```python
from build123d import *

# Parameters (mm, degrees)
SKETCH1_R               = 14.7
SKETCH1_R_2             = 13.4
BOSS_EXTRUDE1_DEPTH     = 7
SKETCH2_W               = 1.6
SKETCH2_H               = 2
BOSS_EXTRUDE2_DEPTH     = 7
CUT_EXTRUDE1_DEPTH      = 22.935815462
CUT_EXTRUDE1_DEPTH_BACK = 22.935815462
SKETCH3_R               = 1.1
SKETCH4_R               = 17.05
SKETCH4_R_2             = 11.5
BOSS_EXTRUDE3_DEPTH     = 2
BOSS_EXTRUDE4_DEPTH     = 2
CUT_EXTRUDE2_REACH      = 27.108
SKETCH6_R               = 1


with BuildPart() as part:
    # Sketch1 → Boss-Extrude1 (new body)
    with BuildSketch(Plane.XY):
        Circle(SKETCH1_R)
        Circle(SKETCH1_R_2, mode=Mode.SUBTRACT)
    extrude(amount=BOSS_EXTRUDE1_DEPTH)

    # Sketch2 → Boss-Extrude2 (add)
    with BuildSketch(Plane.XY):
        with Locations((0, -12.4)):
            Rectangle(SKETCH2_W, SKETCH2_H)
    extrude(amount=BOSS_EXTRUDE2_DEPTH)

    # Sketch3 → Cut-Extrude1 (cut, two sides: drawn at the far end of the back side and taken through both)
    with BuildSketch(Plane(origin=(0, 0, 0), x_dir=(0, 0, -1), z_dir=(1, 0, 0)).offset(-CUT_EXTRUDE1_DEPTH_BACK)):
        with Locations((-3.67, 0)):
            Circle(SKETCH3_R)
    extrude(amount=CUT_EXTRUDE1_DEPTH + CUT_EXTRUDE1_DEPTH_BACK, mode=Mode.SUBTRACT)

    # Sketch4 → Boss-Extrude3 (add)
    with BuildSketch(Plane.XY):
        Circle(SKETCH4_R)
        Circle(SKETCH4_R_2, mode=Mode.SUBTRACT)
    extrude(amount=-BOSS_EXTRUDE3_DEPTH)

    # Sketch5 → Boss-Extrude4 (add)
    with BuildSketch(Plane.XY):
        with BuildLine():
            Line((-6.5, -3), (-3, -3))
            Line((-3, -3), (-3, -11.5))
            Line((-3, -11.5), (3, -11.5))
            Line((3, -11.5), (3, -3))
            Line((3, -3), (6.5, -3))
            ThreePointArc((6.5, -3), (9.5, 0), (6.5, 3))
            Line((6.5, 3), (3, 3))
            Line((3, 3), (3, 11.5))
            Line((3, 11.5), (0, 11.5))
            Line((0, 11.5), (-3, 11.5))
            Line((-3, 11.5), (-3, 3))
            Line((-3, 3), (-6.5, 3))
            ThreePointArc((-6.5, 3), (-9.5, 0), (-6.5, -3))
        make_face()
    extrude(amount=-BOSS_EXTRUDE4_DEPTH)

    # Sketch6 → Cut-Extrude2 (cut, up to next)
    with BuildSketch(Plane.XY, mode=Mode.PRIVATE) as cut_extrude2_sk1:
        Circle(SKETCH6_R)
    cut_extrude2_tool1 = extrude(cut_extrude2_sk1.sketch, amount=-CUT_EXTRUDE2_REACH, mode=Mode.PRIVATE) & part.part
    # Sketch6 → Cut-Extrude2 (cut, up to next)
    with BuildSketch(Plane.XY, mode=Mode.PRIVATE) as cut_extrude2_sk2:
        with Locations((6.5, 0)):
            Circle(SKETCH6_R)
    cut_extrude2_tool2 = extrude(cut_extrude2_sk2.sketch, amount=-CUT_EXTRUDE2_REACH, mode=Mode.PRIVATE) & part.part
    # Sketch6 → Cut-Extrude2 (cut, up to next)
    with BuildSketch(Plane.XY, mode=Mode.PRIVATE) as cut_extrude2_sk3:
        with Locations((-6.5, 0)):
            Circle(SKETCH6_R)
    cut_extrude2_tool3 = extrude(cut_extrude2_sk3.sketch, amount=-CUT_EXTRUDE2_REACH, mode=Mode.PRIVATE) & part.part
    # Sketch6 → Cut-Extrude2 (cut, up to next)
    with BuildSketch(Plane.XY, mode=Mode.PRIVATE) as cut_extrude2_sk4:
        with Locations((0, 8.5)):
            Circle(SKETCH6_R)
    cut_extrude2_tool4 = extrude(cut_extrude2_sk4.sketch, amount=-CUT_EXTRUDE2_REACH, mode=Mode.PRIVATE) & part.part
    # Sketch6 → Cut-Extrude2 (cut, up to next)
    with BuildSketch(Plane.XY, mode=Mode.PRIVATE) as cut_extrude2_sk5:
        with Locations((0, -8.5)):
            Circle(SKETCH6_R)
    cut_extrude2_tool5 = extrude(cut_extrude2_sk5.sketch, amount=-CUT_EXTRUDE2_REACH, mode=Mode.PRIVATE) & part.part
    add(cut_extrude2_tool1.solids().sort_by_distance((0, 0, 0))[0], mode=Mode.SUBTRACT)
    add(cut_extrude2_tool2.solids().sort_by_distance((6.5, 0, 0))[0], mode=Mode.SUBTRACT)
    add(cut_extrude2_tool3.solids().sort_by_distance((-6.5, 0, 0))[0], mode=Mode.SUBTRACT)
    add(cut_extrude2_tool4.solids().sort_by_distance((0, 8.5, 0))[0], mode=Mode.SUBTRACT)
    add(cut_extrude2_tool5.solids().sort_by_distance((0, -8.5, 0))[0], mode=Mode.SUBTRACT)


solid = part.part
```
Source: CAD feature listing. Evaluate the final solid. Frame: model axes, mm. A direction names the side the tool comes from. Give positions to 0.01 mm unless a question says otherwise; leave off trailing zeros. Loops run counter-clockwise (first coordinate to the right, second up) from the corner with the lowest first, then second, coordinate; pieces in that order, holes last. Notation, with made-up numbers: (51, -33.75) - (64, -33.75) arc R31 ccw to (64, -7.75) - close; hole circle Ø2 at (-14.5, -25). An arc over 180 degrees is marked (long way). Use CSV: the item, a comma, the result in double quotes. Start each with the question number.
1. Section C-C (y = 7). Output: boundary loops of the cut face in (x, z).
2. Section A-A (z = 5.5). Output: boundary loops of the cut face in (x, y), then the cut area to 3 significant figures.
3. Section D-D (z = 3.75). Output: boundary loops of the cut face in (x, y), then the cut area to 3 significant figures.
4. Pin query (flat end, axial travel): pin 1 (8 mm diameter, centred on x = 6, y = 4, fed in from +Z); pin 2 (1.5 mm diameter, centred on y = -7, z = -1, fed in from +X); pin 3 (1.6 mm diameter, centred on y = -12, z = 2.5, fed in from -X). Return the tip coordinate at first contact, or that it passes through.
5. Ray query, L1, parallel to Y at x = 0, z = -0.85; L2, parallel to X at y = 0, z = 2.25; L3, parallel to X at y = -11.5, z = 3.5. Return the intervals inside material, ascending.
6. Section B-B (x = 11). Output: boundary loops of the cut face in (y, z), then the cut area to 3 significant figures.
7. Draft query along Y for faces 1 (the cylindrical face through (5.7, -0.6, -1)), 2 (the cylindrical face through (14.02, 4.42, 3.45)), 3 (the flat face through (0, -13, 7)). Return one class per face: +Y half, -Y half, draft (parallel to the pull), parting line (faces both ways), or undercut.
8. Reachability of faces 4 (the flat face through (3, 7, -1)), 5 (the flat face through (0, -11.4, 3)), 6 (the cylindrical face through (-14.04, 0.33, 2.62)) from +Z, -Z, +X, -X, +Y, -Y: full face, straight path, thin tool, end or side. Return the list, or none.
Response:
1,outline,"(-15.55, -2) - (-9.12, -2) - (-9.12, 0) - (-11.43, 0) - (-11.43, 7) - (-12.93, 7) - (-12.93, 0) - (-15.55, 0) - close; (-3, -2) - (3, -2) - (3, 0) - (-3, 0) - close; (9.12, -2) - (15.55, -2) - (15.55, 0) - (12.93, 0) - (12.93, 7) - (11.43, 7) - (11.43, 0) - (9.12, 0) - close"
2,outline,"circle Ø29.4 at (0, 0); hole (-0.8, -13.38) - (-0.8, -11.4) - (0.8, -11.4) - (0.8, -13.38) arc R13.4 ccw (long way) to start"
2,area,"118 mm²"
3,outline,"(-14.66, -1.1) arc R14.7 ccw to (14.66, -1.1) - (13.36, -1.1) arc R13.4 cw to (0.8, -13.38) - (0.8, -11.4) - (-0.8, -11.4) - (-0.8, -13.38) arc R13.4 cw to (-13.36, -1.1) - close; (-14.66, 1.1) - (-13.36, 1.1) arc R13.4 cw to (13.36, 1.1) - (14.66, 1.1) arc R14.7 ccw to start"
3,area,"112 mm²"
4,pin 1,"z = 0"
4,pin 2,"x = 15.86"
4,pin 3,"x = -9.52"
5,L1,"-17.05 to -9.5, -7.5 to -1, 1 to 7.5, 9.5 to 17.05"
5,L2,"-14.7 to -13.4, 13.4 to 14.7"
5,L3,"-9.16 to -6.88, -0.8 to 0.8, 6.88 to 9.16"
6,outline,"(-13.03, -2) - (-3.35, -2) - (-3.35, 0) - (-7.65, 0) - (-7.65, 7) - (-9.75, 7) - (-9.75, 0) - (-13.03, 0) - close; (3.35, -2) - (13.03, -2) - (13.03, 0) - (9.75, 0) - (9.75, 7) - (7.65, 7) - (7.65, 0) - (3.35, 0) - close"
6,area,"68.1 mm²"
7,face 1,"undercut"
7,face 2,"parting line"
7,face 3,"draft"
8,face 4,"+Z, -Z"
8,face 5,"+Z"
8,face 6,"+X, -X"
